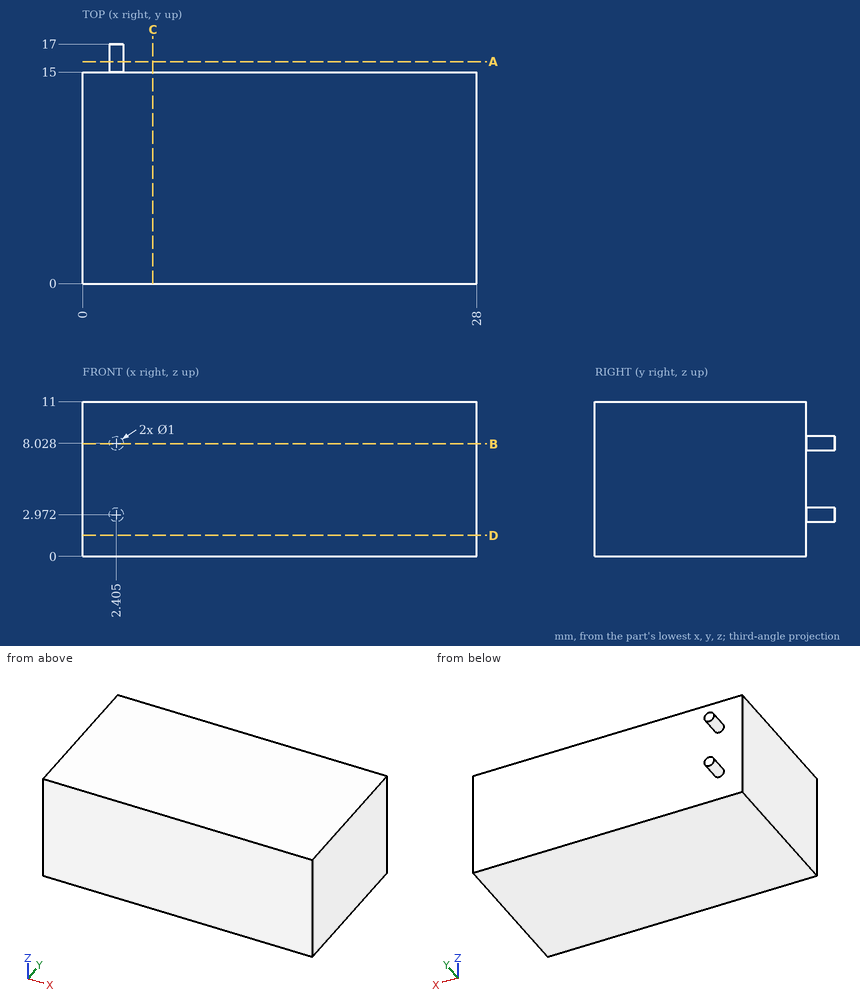
Geometry: see drawing. Coordinates: mm, zero at the bounding-box minimum. Round coordinates to 2 decimals unless told otherwise and drop trailing zeros. Loops run counter-clockwise (first coordinate to the right, second up) from the corner with the lowest first, then second, coordinate; pieces in that order, holes last. Notation, with made-up numbers: M 29.5,9.25 L 48.5,9.25 A16 cw 48.5,34.25 Z; hole C -0.75,-9.5 d8. An arc over 180 degrees is marked long. Use a Markdown table: item, result. Add a question column.
1. Cut plane D-D, the plane z = 1.5. Output: boundary loops of the cut face in (x, y).
2. Cut plane C-C, the plane x = 5. Output: boundary loops of the cut face in (y, z).
3. Cut plane B-B, the plane z = 8. Output: boundary loops of the cut face in (x, y) (1 decimal), and give its area (3 significant figures).
4. Cut plane A-A, the plane y = 15.75. Output: boundary loops of the cut face in (x, z) (1 decimal).
5. Ray query, line 1 along Y through (x, z) = (1.5, 3.5); line 2 along X through (y, z) = (15.25, 3.25). Return the intervals inside material, ascending. Write a range as [from, to].
6. Contact query for flat-ended pins moving along their axis: pin 1 (2 mm diameter, centred on y = 8.5, z = 9.5, fed in from -X); pin 2 (5.5 mm diameter, centred on x = 11.5, z = 4.5, fed in from +Y). Output: stop coordinate, or through.
Solution:
| question | item | result |
|---|---|---|
| 1 | outline | M 0,0 L 28,0 L 28,15 L 0,15 Z |
| 2 | outline | M 0,0 L 15,0 L 15,11 L 0,11 Z |
| 3 | outline | M 0,0 L 28,0 L 28,15 L 2.9,15 L 2.9,17 L 1.9,17 L 1.9,15 L 0,15 Z |
| 3 | area | 422 mm2 |
| 4 | outline | C 2.4,3 d1; C 2.4,8 d1 |
| 5 | line 1 | y = [0, 15] |
| 5 | line 2 | x = [1.99, 2.82] |
| 6 | pin 1 | stops at x = 0 |
| 6 | pin 2 | stops at y = 15 |
